The figure shows three views and two pictorial views of one solid part (mm, origin at its lowest corner). Answer the questions. A direction names the side the tool comes from. Give positions to 0.01 mm unless a question says otherwise; leave off trailing zeros. Loops run counter-clockwise (first coordinate to the right, second up) from the corner with the lowest first, then second, coordinate; pieces in that order, holes last. Notation, with made-up numbers: (64, 41) - (112, 41) arc R14 cw to (112, 50) - close; hole circle Ø8 at (63, 33.25). An arc over 180 degrees is marked (long way). Write each question's results on one line, items separated by ' | '.
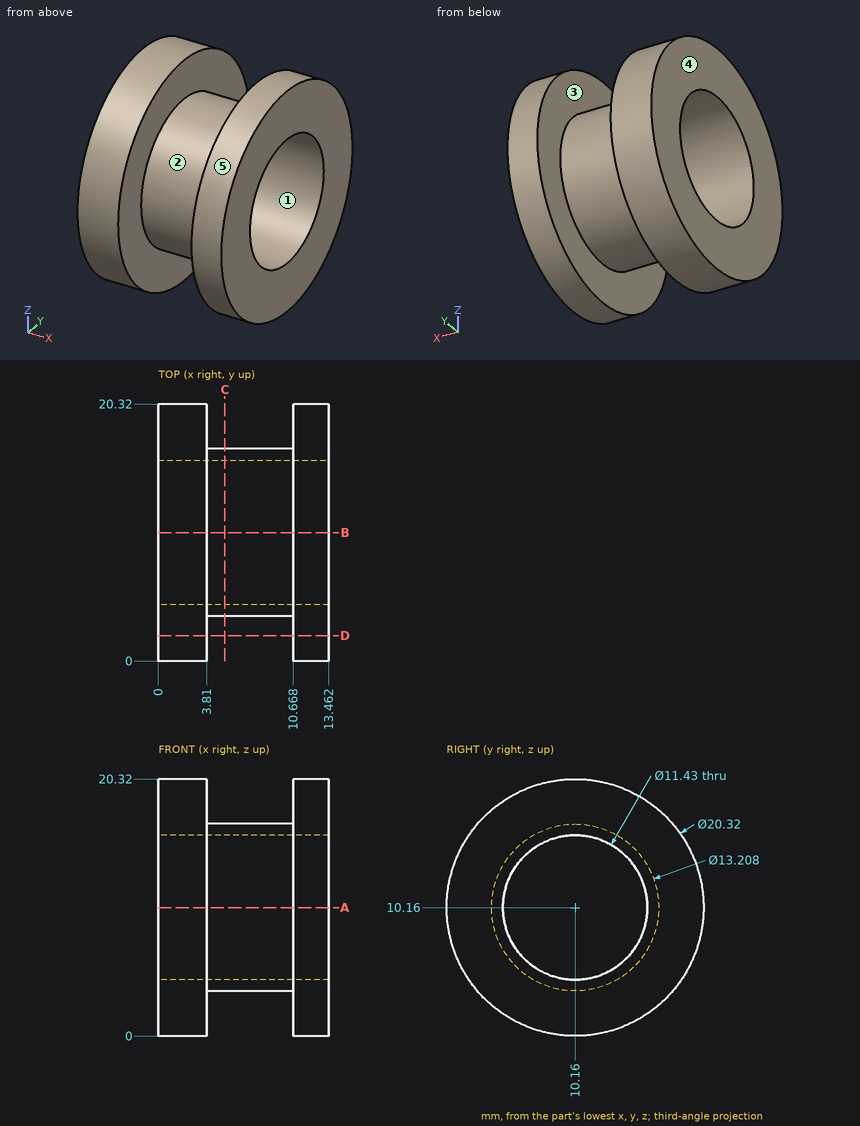
Item 1: For the marked faces 1 and 2, determine the directions among +Z, -Z, +X, -X, +Y, -Y from which every point of the face is accessible in a straight line to the end or side of a thin tool.
Values found:
face 1: +X, -X | face 2: none
Item 2: Flat-ended cylindrical pins translate along their axes: P1, Ø6, axis at x = 6, z = 12, coming from the +Y side; P2, Ø4, axis at x = 11, y = 13.5, coming from the -Z side; P3, Ø1, axis at x = 7, z = 7.5, coming from the -Y side; P4, Ø5, axis at x = 1.5, y = 2.5, coming from the +Z side. Find the tip coordinate at first contact, or state that the pin passes through.
Values found:
P1: stops at y = 20.32 | P2: stops at z = 0.09 | P3: stops at y = 3.92 | P4: stops at z = 18.91
Item 3: A cutting plane is placed at D-D, the plane y = 2. Determine the outline of the cut face in (x, z), plus the area to 3 significant figures.
Values found:
outline: (0, 4.11) - (3.81, 4.11) - (3.81, 16.21) - (0, 16.21) - close; (10.67, 4.11) - (13.46, 4.11) - (13.46, 16.21) - (10.67, 16.21) - close | area: 79.9 mm²
Item 4: A cutting plane is placed at A-A, the plane z = 10.16. Determine the outline of the cut face in (x, y) (3 decimals).
Values found:
outline: (0, 0) - (3.81, 0) - (3.81, 3.556) - (10.668, 3.556) - (10.668, 0) - (13.462, 0) - (13.462, 4.445) - (0, 4.445) - close; (0, 15.875) - (13.462, 15.875) - (13.462, 20.32) - (10.668, 20.32) - (10.668, 16.764) - (3.81, 16.764) - (3.81, 20.32) - (0, 20.32) - close
Item 5: Find the intervals of material crossed by line 1 along X through (y, z) = (2.5, 16.5); line 2 along Y through (x, z) = (12.5, 10.25); line 3 along Y through (x, z) = (4.25, 10.16) (3 decimals), in increasing order. Write a range as [from, to].
Values found:
line 1: x = [0, 3.81], [10.67, 13.46] | line 2: y = [0, 4.45], [15.87, 20.32] | line 3: y = [3.556, 4.445], [15.875, 16.764]
Item 6: For a pull along X with two mould halves and no side action, classify the marked faces 3, 4 and 5 as released by +X, released by -X, zero draft, split by the parting line, or undercut.
Values found:
face 3: undercut | face 4: released by -X | face 5: zero draft
Item 7: A cutting plane is placed at C-C, the plane x = 5.25. Determine the outline of the cut face in (y, z) (3 decimals).
Values found:
outline: circle Ø13.208 at (10.16, 10.16); hole circle Ø11.43 at (10.16, 10.16)
